Read the model definition and answer for the solid it produces. Units are mm, in the model's axes. A direction names the side the tool comes from. Coordinates: 2 decimals unless noted, no trailing zeros. Write each loop counter-clockwise with the first axis right and the second up, starting at its lowest first coordinate (ties: lowest second). Pieces come first, ordered by that corner, then holes. Notation, with made-up numbers: (59, -24.75) - (74, -24.75) arc R31 cw to (74, 8.25) - close; hole circle Ø2 at (88, -17.5). An arc over 180 degrees is marked (long way). Use a Markdown table: item, result.
from build123d import *

# Parameters (mm, degrees)
SKETCH1_W           = 25
SKETCH1_H           = 95
BOSS_EXTRUDE1_DEPTH = 10
SKETCH2_R           = 10
CUT_EXTRUDE1_DEPTH  = 7.5
SWEEP1_PROFILE_R    = 0.5


with BuildPart() as part:
    # Sketch1 → Boss-Extrude1 (new body, symmetric)
    with BuildSketch(Plane.XY):
        with Locations((-37.921146953, 2.311827957)):
            Rectangle(SKETCH1_W, SKETCH1_H)
    extrude(amount=BOSS_EXTRUDE1_DEPTH, both=True)

    # Sketch2 → Cut-Extrude1 (cut, symmetric)
    with BuildSketch(Plane.XY):
        with Locations((-37.921146953, 49.811827957)):
            Circle(SKETCH2_R)
    extrude(amount=CUT_EXTRUDE1_DEPTH, both=True, mode=Mode.SUBTRACT)

    # Sweep1: sweep along a path in Sketch4
    with BuildLine(Plane.ZY.offset(37.921146953)) as sweep1_path:
        Line((-10, 50.309963159), (10, 50.309963159))
    # Sweep1 profile (on start of the path) → Sweep1 (sweep)
    with BuildSketch(Plane(origin=(-37.921146953, 50.309963159, -10), x_dir=(1, 0, 0), z_dir=(0, 0, 1))):
        Circle(SWEEP1_PROFILE_R)
    sweep(path=sweep1_path.line)


solid = part.part
(1) The mould has two halves that part along X. Classify faces 1 (the flat face through (-50.421, 2, 0)), 2 (the flat face through (-38, 46, -7.5)), 3 (the flat face through (-25.421, 2, 0)), 4 (the flat face through (-38, 3, -10)): pulls with the +X half, pulls with the -X half, needs draft (parallel to the pull), parting line crosses it, or undercut.
Report:
| item | result |
|---|---|
| face 1 | pulls with the -X half |
| face 2 | undercut |
| face 3 | pulls with the +X half |
| face 4 | needs draft |
(2) This flat-tipped pin is pushed along its axis until it touches: P1, Ø5, axis at x = -46, z = 2, coming from the +Y side. Where does it stop, or does it pass through?
Report:
| item | result |
|---|---|
| P1 | stops at y = 49.81 |
(3) A cutting plane is placed at A-A, the plane x = -39.75. Write down the section's boundary in (y, z).
Report:
| item | result |
|---|---|
| outline | (-45.19, -10) - (49.81, -10) - (49.81, -7.5) - (39.98, -7.5) - (39.98, 7.5) - (49.81, 7.5) - (49.81, 10) - (-45.19, 10) - close |
(4) A cutting plane is placed at C-C, the plane x = -45. Write down the section's boundary in (y, z).
Report:
| item | result |
|---|---|
| outline | (-45.19, -10) - (49.81, -10) - (49.81, -7.5) - (42.75, -7.5) - (42.75, 7.5) - (49.81, 7.5) - (49.81, 10) - (-45.19, 10) - close |
(5) A cutting plane is placed at B-B, the plane z = 5.75. Write down the section's boundary in (x, y), and give its area (3 significant figures).
Report:
| item | result |
|---|---|
| outline | (-50.42, -45.19) - (-25.42, -45.19) - (-25.42, 49.81) - (-27.92, 49.81) arc R10 cw to (-47.92, 49.81) - (-50.42, 49.81) - close; circle Ø1 at (-37.92, 50.31) |
| area | 2,220 mm² |
(6) For faces 5 (the flat face through (-38, -45.188, 0)), 6 (the flat face through (-38, 46, 7.5)), determine the directions among +Z, -Z, +X, -X, +Y, -Y from which every point of the face is accessible in a straight line to the end or side of a thin tool.
Report:
| item | result |
|---|---|
| face 5 | +Z, -Z, +X, -X, -Y |
| face 6 | none |
(7) Straight lines are drawn through the part: L1, parallel to Y at x = -27.5, z = 4.75; L2, parallel to X at y = 43, z = -7.25; L3, parallel to Y at x = -36.25, z = 5.25. For each, find the intervals that lie inside material, in ascending order.
Report:
| item | result |
|---|---|
| L1 | y = -45.19 to 49.81 |
| L2 | x = -50.42 to -45.24, -30.6 to -25.42 |
| L3 | y = -45.19 to 39.95 |
